Study the drawing (mm; zero at the part's minimum x, y, z) and answer. Give positions to 0.01 mm unless a question says otherwise; leave off trailing zeros. Order: outer loops, then holes, each group sorted by start corner. A loop starts at its lowest first (then second) coordinate and runs counter-clockwise, first axis right, second up. Notation, with made-up numbers: (10, 8.5) - (63, 8.5) arc R34 cw to (63, 44.5) - close; hole circle Ø4 at (-12, 5.5). An arc over 180 degrees is marked (long way). Return JSON: item names as keys, results as strings.
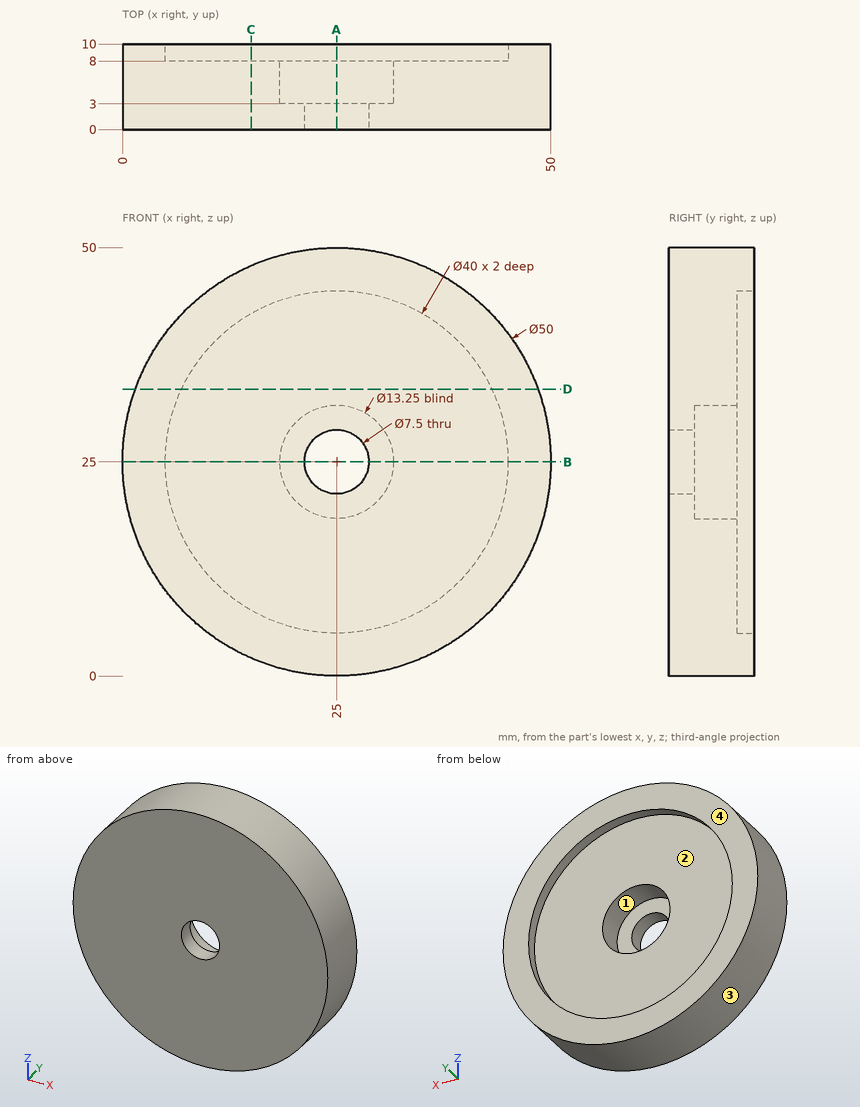
Q1. A cutting plane is placed at A-A (x = 25). Write down the section's boundary in (y, z) (3 decimals).
Values:
{"outline": "(0, 0) - (10, 0) - (10, 5) - (8, 5) - (8, 18.375) - (3, 18.375) - (3, 21.25) - (0, 21.25) - close; (0, 28.75) - (3, 28.75) - (3, 31.625) - (8, 31.625) - (8, 45) - (10, 45) - (10, 50) - (0, 50) - close"}
Q2. Determine the mould class of the marked faces 1, 2, 3 and 4 for opening direction Z: released by +Z, released by -Z, zero draft, split by the parting line, or undercut.
Values:
{"face 1": "undercut", "face 2": "undercut", "face 3": "split by the parting line", "face 4": "zero draft"}
Q3. Given pin 1 (5 mm diameter, centred on x = 36, y = 3, fed in from -Z); pin 2 (6.5 mm diameter, centred on x = 23, z = 27, fed in from +Y); pin 3 (5 mm diameter, centred on x = 7.5, y = 5, fed in from -Z); pin 4 (7 mm diameter, centred on x = 25, z = 25, fed in from -Y), each flat-ended and moving along its own axis, determine where each tip first touches the part or whether it passes through.
Values:
{"pin 1": "stops at z = 1.49", "pin 2": "stops at y = 3", "pin 3": "stops at z = 5", "pin 4": "passes through"}
Q4. Consider L1, parallel to X at y = 0.9, z = 25; L2, parallel to Z at x = 25, y = 8.9; L3, parallel to Z at x = 25, y = 4.45 (3 decimals). Determine where each line is inside the solid, lowest interval first.
Values:
{"L1": "x = 0 to 21.25, 28.75 to 50", "L2": "z = 0 to 5, 45 to 50", "L3": "z = 0 to 18.375, 31.625 to 50"}
Q5. A cutting plane is placed at D-D (z = 33.5). Write down the section's boundary in (x, y), and give its area (3 significant figures).
Values:
{"outline": "(1.49, 0) - (48.51, 0) - (48.51, 10) - (43.1, 10) - (43.1, 8) - (6.9, 8) - (6.9, 10) - (1.49, 10) - close", "area": "398 mm²"}
Q6. A cutting plane is placed at B-B (z = 25). Write down the section's boundary in (x, y) (3 decimals).
Values:
{"outline": "(0, 0) - (21.25, 0) - (21.25, 3) - (18.375, 3) - (18.375, 8) - (5, 8) - (5, 10) - (0, 10) - close; (28.75, 0) - (50, 0) - (50, 10) - (45, 10) - (45, 8) - (31.625, 8) - (31.625, 3) - (28.75, 3) - close"}
Q7. A cutting plane is placed at C-C (x = 15). Write down the section's boundary in (y, z), and give its area (3 significant figures).
Values:
{"outline": "(0, 2.09) - (10, 2.09) - (10, 7.68) - (8, 7.68) - (8, 42.32) - (10, 42.32) - (10, 47.91) - (0, 47.91) - close", "area": "389 mm²"}
